Geometry check sheet. Reference: the model listing, model coordinates, mm. Face numbers are marked on the shaded views. A direction names the side the tool comes from. Round coordinates to 2 decimals unless told otherwise and drop trailing zeros. Order: outer loops, then holes, each group sorted by start corner. A loop starts at its lowest first (then second) coordinate and runs counter-clockwise, first axis right, second up. Notation, with made-up numbers: (-35, 80) - (9, 80) arc R21 cw to (9, 115) - close; hole circle Ø3 at (-40, 1). An arc over 180 degrees is marked (long way). One line per question, with ' | ' between items. Start each with the question number.
Q1. Tool access check on the marked faces 1, 2 and 3. Record the directions out of +Z, -Z, +X, -X, +Y, -Y that give a thin tool (end or side, any length) a straight path to the whole face; none if there is none.
Q2. Material ranges on line 1 along Z through (x, y) = (149, -6.5); line 2 along Y through (x, z) = (169.5, 42); line 3 along X through (y, z) = (-96, 59), recorded low to high.
Q3. Gauge pin test, flat end, axial feed: P1, Ø8, axis at x = 121, y = -67.5, coming from the +Z side. Record the tip position at first contact, or that the pin passes through.
Q4. Sectioned sample at B-B, the plane z = 20. Enter the section's corners in (x, y), then the cut area to 3 significant figures.
Q5. Sectioned sample at C-C, the plane y = -111.5. Enter the section's corners in (x, z), then the cut area to 3 significant figures.
Q6. Sectioned sample at A-A, the plane x = 173. Enter the section's corners in (y, z), then the cut area to 3 significant figures.
Q7. Sectioned sample at D-D, the plane x = 106. Enter the section's corners in (y, z).
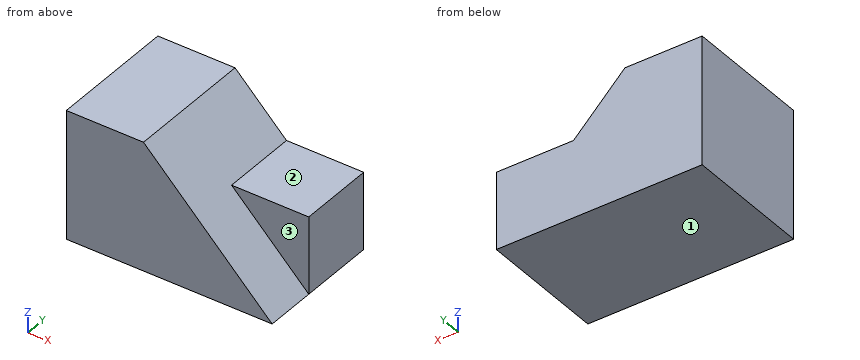
```python
from build123d import *

# Parameters (mm, degrees)
F1_DEPTH = 127
F2_DEPTH = 76.2


with BuildPart() as f1:
    # F0 (on Front) → F1 (new body)
    with BuildSketch(Plane.XZ):
        Polygon((0, 127), (0, 0), (203.2, 0), (127, 76.2), (76.2, 127), align=None)
    extrude(amount=F1_DEPTH)

    # F0 (on Front) → F2 (join)
    with BuildSketch(Plane.XZ):
        Polygon((127, 76.2), (203.2, 0), (203.2, 76.2), align=None)
    extrude(amount=F2_DEPTH)


solid = f1.part
```
Determined:
1) face 1: -Z, +X, -X, +Y, -Y | face 2: +Z, +X, +Y, -Y | face 3: +Z, +X, -Y
2) line 1: z = 0 to 76.2 | line 2: y = -76.2 to 0 | line 3: x = 0 to 144.2
3) P1: stops at z = 86.2
4) outline: (0, -127) - (183.2, -127) - (183.2, -76.2) - (203.2, -76.2) - (203.2, 0) - (0, 0) - close | area: 24,800 mm2
5) outline: (0, 0) - (203.2, 0) - (76.2, 127) - (0, 127) - close | area: 17,700 mm2
6) outline: (-127, 0) - (0, 0) - (0, 76.2) - (-76.2, 76.2) - (-76.2, 30.2) - (-127, 30.2) - close | area: 7,340 mm2
7) outline: (-127, 0) - (0, 0) - (0, 97.2) - (-127, 97.2) - close
